```python
from build123d import *

# Parameters (mm, degrees)
F0_R     = 1.5
F0_R_2   = 2.1
F1_DEPTH = 6
F2_R     = 3.98
F3_DEPTH = 26
F4_R     = 1.5
F5_DEPTH = 4
F6_SIZE  = 3.99999


# Not quite as in the source:
# - a fillet or chamfer is up to 0.001 mm smaller than in the source, because OpenCascade refuses the exact size


with BuildPart() as f1:
    # F0 (on Top) → F1 (new body)
    with BuildSketch(Plane.XY):
        with BuildLine():
            Line((4.5, 0), (4.5, 3.9686269666))
            ThreePointArc((4.5, 3.9686269666), (0, 6), (-4.5, 3.9686269666))
            Line((-4.5, 3.9686269666), (-4.5, 0))
            Line((-4.5, 0), (-4.5, -5.813701588))
            Line((-4.5, -5.813701588), (-15.143203234, -16.4569048219))
            ThreePointArc((-15.143203234, -16.4569048219), (-15.1189316865, -21.3823807428), (-10.1934557657, -21.4066522902))
            Line((-10.1934557657, -21.4066522902), (4.5, -7))
            Line((4.5, -7), (4.5, 0))
        make_face()
        with Locations((-12.6691633098, -18.9323580438)):
            Circle(F0_R, mode=Mode.SUBTRACT)
        Circle(F0_R_2, mode=Mode.SUBTRACT)
    extrude(amount=F1_DEPTH)

    # F2 (on face) → F3 (join)
    with BuildSketch(Plane(origin=(5.7049735344, -5.8185465008, 0), x_dir=(0.7140411723, 0.7001037097, 0), z_dir=(0.7001037097, -0.7140411723, 0))):
        with Locations((-11.9764822387, -0.39)):
            Circle(F2_R)
    extrude(amount=F3_DEPTH)

    # F4 (on face) → F5 (join)
    with BuildSketch(Plane(origin=(0, 0, 0), x_dir=(1, 0, 0), z_dir=(0, 0, -1))):
        with BuildLine():
            ThreePointArc((-10.1934557657, 21.4066522902), (-15.1189316865, 21.3823807428), (-15.143203234, 16.4569048219))
            Line((-15.143203234, 16.4569048219), (-4.5, 5.813701588))
            Line((-4.5, 5.813701588), (4.5, 7))
            Line((4.5, 7), (-10.1934557657, 21.4066522902))
        make_face()
        with Locations((-12.6691633098, 18.9323580438)):
            Circle(F4_R, mode=Mode.SUBTRACT)
    extrude(amount=F5_DEPTH)

    # F6 (size 4 in the source; OpenCascade refuses exactly that, so slightly less here)
    f6_edges = [f1.edges().sort_by_distance(p)[0] for p in [
        (0, -6.406851, -4),
    ]]
    chamfer(f6_edges, length=F6_SIZE)


solid = f1.part
```
CAD build for the part. Positions are in the model's coordinates, mm. A direction names the side the tool comes from. Round coordinates to 2 decimals unless told otherwise and drop trailing zeros. Write each loop counter-clockwise with the first axis right and the second up, starting at its lowest first coordinate (ties: lowest second). Pieces come first, ordered by that corner, then holes. Notation, with made-up numbers: (13, -29) - (21, -29) arc R20 ccw to (21, -18) - close; hole circle Ø9 at (-24.75, -7). An arc over 180 degrees is marked (long way). Write item = value, one per line. Start each with the question number.
Q1. Band-saw the part on C-C (y = -18). Count the separate pieces of the cut face and the enclosed holes in it, then the cut area to 3 significant figures.
Q2. Band-saw the part on D-D (x = -7.5). Give the cut face in (y, z), then the cut area to 3 significant figures.
Q3. Mould opens along X. For faces 4 (the flat face through (2, -2, 0)), 5 (the cylindrical face through (-12.86, -20.42, 1.07)), 6 (the cylindrical face through (0, 6, 3)) say: pulls with the +X half, pulls with the -X half, needs draft (parallel to the pull), parting line crosses it, or undercut.
Q4. Drop flat-ended pins along their axis: pin 1 (3 mm diameter, centred on x = -10.5, z = -2, fed in from -Y); pin 2 (5 mm diameter, centred on y = 0.5, z = 3.5, fed in from +X); pin 3 (1.5 mm diameter, centred on y = -29, z = 2.5, fed in from +X). Give the stop position or say it passes through.
Q5. Band-saw the part on B-B (z = 3). Give the cut face in (x, y), then the cut area to 3 significant figures.
Q6. Band-saw the part on A-A (y = 0). Give the cut face in (x, z), then the cut area to 3 significant figures.
Q7. Probe L1, parallel to Y at x = 0, z = 4.25; L2, parallel to Z at x = -0.5, y = -5; L3, parallel to Z at x = -10, y = -19.5. List the from-to ranges inside material, lowest first. Write a range as from..to.
Q8. Which spindle directions (+Z, -Z, +X, -X, +Y, -Y) get a long thin tool onto all of the face, cutting with end or side? Do faces 1 (the flat face through (4.5, -2, 3)), 2 (the flat face through (-4.5, -1, 3)), 3 (the flat face through (-10, -16, -4)). Say none if no direction does.
Answers below:
q1.separate_pieces = 3
q1.enclosed_holes = 0
q1.area = 139 mm2
q2.outline = (-18.77, -4) - (-9.45, -4) - (-8.81, -3.37) - (-8.81, 6) - (-18.77, 6) - close
q2.area = 99.3 mm2
q3.face_4 = needs draft
q3.face_5 = undercut
q3.face_6 = parting line crosses it
q4.pin_1 = -22.35
q4.pin_2 = 4.5
q4.pin_3 = 16.67
q5.outline = (-15.14, -16.46) arc R3.5 ccw to (-10.19, -21.41) - (-4.34, -15.66) - (13.87, -34.23) - (16.84, -31.31) - (-1.36, -12.74) - (4.5, -7) - (4.5, 3.97) arc R6 ccw to (-4.5, 3.97) - (-4.5, -5.81) - close; hole circle Ø3 at (-12.67, -18.93); hole circle Ø4.2 at (0, 0)
q5.area = 339 mm2
q6.outline = (-4.5, 0) - (-2.1, 0) - (-2.1, 6) - (-4.5, 6) - close; (2.1, 0) - (4.5, 0) - (4.5, 6) - (2.1, 6) - close
q6.area = 28.8 mm2
q7.L1 = -11.41..-2.1, 2.1..6
q7.L2 = 0..6
q7.L3 = -4..6
q8.face_1 = +Z, -Z, +X, +Y
q8.face_2 = +Z, -Z, -X, +Y
q8.face_3 = -Z, -X, +Y
